Autodesk Inventor part; units mm, degrees
ref_plane "YZ Plane" through (0, 0, 0) normal (1, 0, 0) x (0, 1, 0)
ref_plane "XZ Plane" through (0, 0, 0) normal (0, 1, 0) x (-1, 0, 0)
ref_plane "XY Plane" through (0, 0, 0) normal (0, 0, 1) x (1, 0, 0)
sketch "Boceto1" plane through (0, 0, 0) normal (0, 1, 0) x (-1, 0, 0)
  line L0 (0, 0) -> (200, 0)
  line L1 (200, 0) -> (200, -200)
  line L2 (200, -200) -> (0, -200)
  line L3 (0, -200) -> (0, 0)
  dimension "d0" = 200
  dimension "d1" = 200
extrude "Extrusión1" add sketch "Boceto1" along normal blind 5
sketch "Boceto2" plane through (0, 5, 0) normal (0, 1, 0) x (1, 0, 0)
  line L0 (-130, 70) -> (-70, 70)
  line L1 (-70, 70) -> (-70, 130)
  line L2 (-70, 130) -> (-130, 130)
  line L3 (-130, 130) -> (-130, 70)
  line L4 (-200, 200) -> (-200, 0)
  line L5 (-200, 0) -> (0, 0)
  point P0 (-130, 100)
  dimension "d4" = 60
  dimension "d5" = 60
  dimension "d6" = 70
  dimension "d7" = 70
extrude "Extrusión2" add sketch "Boceto2" along normal blind 2000
sketch "Boceto3" plane through (-130, 5, -130) normal (-1, 0, 0) x (0, 0, 1)
  line L0 (0, 0) -> (0, 2000)
  line L1 (0, 2000) -> (60, 2000)
  line L2 (60, 2000) -> (60, 1940)
  line L3 (60, 1940) -> (0, 1940)
  line L4 (0, 1940) -> (0, 2000)
  point P0 (130, -5)
  dimension "d10" = 60
  dimension "d11" = 60
extrude "Extrusión3" add sketch "Boceto3" along normal blind 600
sketch "Boceto4" plane through (-130, 5, -70) normal (0, 0, 1) x (1, 0, 0)
  arc A0 (-540, 1914) -> (-590, 1914) centre (-565, 1914) ccw
  line L0 (-600, 1940) -> (-600, 2000)
  line L1 (0, 1940) -> (-600, 1940)
  arc A1 (-537.5, 1914) -> (-592.5, 1914) centre (-565, 1914) ccw
  line L2 (-592.5, 1914) -> (-590, 1914)
  line L3 (-540, 1914) -> (-537.5, 1914)
  point P0 (130, -5)
  dimension "d14" = 50
  dimension "d15" = 35
  dimension "d16" = 26
  dimension "d17" = 55
extrude "Extrusión4" add sketch "Boceto4" against normal blind 60
sketch "Boceto5" plane through (0, 0, 0) normal (0, -1, 0) x (1, 0, 0)
  line L0 (0, 0) -> (0, -200)
  line L1 (0, -100) -> (-200, -100)
  line L2 (-200, -200) -> (-200, 0)
  line L3 (0, -200) -> (-200, -200)
  line L4 (-100, -200) -> (-100, 0)
  line L5 (-200, 0) -> (0, 0)
  circle A0 centre (-100, -175) radius 9.25
  circle A1 centre (-175, -100) radius 9.25
  circle A2 centre (-100, -25) radius 9.25
  circle A3 centre (-25, -100) radius 9.25
  point P0 (-100, -100)
  point P1 (-100, -100)
  point P2 (-100, -100)
  point P3 (-100, -100)
  dimension "d20" = 18.5
  dimension "d21" = 75
  dimension "d24" = 360
extrude "Extrusión5" cut sketch "Boceto5" against normal blind 10 contours A3 L1 | L1 A3 | A2 L4 | L4 A2 | A0 L4 | L4 A0 | A1 L1 | L1 A1
properties part number "Sriel"
Geometry: final body of the model. Coordinates: model frame, mm. A direction names the side the tool comes from. Round coordinates to 2 decimals unless told otherwise and drop trailing zeros. Order: outer loops, then holes, each group sorted by start corner. A loop starts at its lowest first (then second) coordinate and runs counter-clockwise, first axis right, second up. Notation, with made-up numbers: (70, 85) -> (98, 85) arc R9 ccw to (98, 95) -> close; hole circle Ø8 at (-27.75, 84). An arc over 180 degrees is marked (long way). Use one line per item in the form item = value.
(1) First-contact query: pin 1 Ø1.5 at (x, z) = (-325.5, -121.5) entering from -Y; pin 2 Ø2 at (x, z) = (-669, -112.5) entering from -Y; pin 3 Ø16.5 at (x, z) = (-100, -175) entering from +Y; pin 4 Ø2.5 at (y, z) = (3, -130.5) entering from -X. Flat tips, straight axial feed; report the tip coordinate or a pass-through.
Results list:
pin_1 = 1945
pin_2 = 1919
pin_3 = through
pin_4 = -200
(2) Draft query along X for faces 1 (the face through (-129.6, 1231.9, -70)), 2 (the face through (-694.45, 1943.994, -99.58)), 3 (the face through (-70, 991, -100)), 4 (the face through (-404, 1945, -100)). Return one class per face: pulls with the +X half, pulls with the -X half, needs draft (parallel to the pull), parting line crosses it, or undercut.
Results list:
face_1 = needs draft
face_2 = undercut
face_3 = pulls with the +X half
face_4 = undercut
(3) Access query for faces 5 (the face through (-395, 2005, -100)), 6 (the face through (-105, 1223, -130)). Directions: +Z, -Z, +X, -X, +Y, -Y. A direction counts if a zero-diameter tool reaches every point of the face in a straight line with its end or side. Return the directions, or none.
Results list:
face_5 = +Z, -Z, +X, -X, +Y
face_6 = -Z, +X, -X, +Y
(4) Section A-A on z = -148.5. Return loops of the section in (x, y).
Results list:
outline = (-200, 0) -> (0, 0) -> (0, 5) -> (-200, 5) -> close
(5) Section B-B on y = 870.5. Return loops of the section in (x, z).
Results list:
outline = (-130, -130) -> (-70, -130) -> (-70, -70) -> (-130, -70) -> close
(6) Ray query, probe 1 along Z at (x, y) = (-100, 4.05); probe 2 along X at (y, z) = (3.25, -25). Return the intervals inside material, ascending. Write a range as [from, to].
Results list:
probe_1 = [-200, -184.25], [-165.75, -34.25], [-15.75, 0]
probe_2 = [-200, -109.25], [-90.75, 0]
